Read the model definition and answer for the solid it produces. Units are mm, in the model's axes. A direction names the side the tool comes from. Coordinates: 2 decimals unless noted, no trailing zeros. Order: outer loops, then holes, each group sorted by start corner. A loop starts at its lowest first (then second) coordinate and runs counter-clockwise, first axis right, second up. Notation, with made-up numbers: (43, 84) -> (90, 84) arc R14 ccw to (90, 92) -> close; hole circle Ø2 at (34, 20.5). An arc over 180 degrees is marked (long way). Answer in a Markdown table with one row per item.
from build123d import *

# Parameters (mm, degrees)
CROQUIS1_W              = 19
CROQUIS1_H              = 15
SALIENTE_EXTRUIR1_DEPTH = 7
CROQUIS2_W              = 8
CROQUIS2_H              = 8
CROQUIS2_R              = 1
SALIENTE_EXTRUIR2_DEPTH = 4.9
CROQUIS3_W              = 19
CROQUIS3_H              = 3.8
CORTAR_EXTRUIR1_DEPTH   = 37.9
CROQUIS4_R              = 1
CORTAR_EXTRUIR2_DEPTH   = 51.9


with BuildPart() as part:
    # Croquis1 → Saliente-Extruir1 (new body)
    with BuildSketch(Plane(origin=(0, 0, 0), x_dir=(1, 0, 0), z_dir=(0, 1, 0))):
        Polygon((16.592354246, -24.663454956), (16.592354246, 24.436543518), (8.592354246, 24.436543518), (8.592354246, 14.886544281), (-10.407645754, 14.886544281), (-10.407645754, 24.436543518), (-18.407645754, 24.436543518), (-18.407645754, -24.663454956), (-10.407645754, -24.663454956), (-10.407645754, -15.113455719), (8.592354246, -15.113455719), (8.592354246, -24.663454956), align=None)
        with Locations((-0.907645754, -0.113455719)):
            Rectangle(CROQUIS1_W, CROQUIS1_H, mode=Mode.SUBTRACT)
    extrude(amount=SALIENTE_EXTRUIR1_DEPTH)

    # Croquis2 → Saliente-Extruir2 (add)
    with BuildSketch(Plane(origin=(0, 7, 0), x_dir=(1, 0, 0), z_dir=(0, 1, 0))):
        with Locations((-14.407645754, -0.113455719)):
            Rectangle(CROQUIS2_W, CROQUIS2_H)
        with Locations((-14.407645754, -0.113455719)):
            Circle(CROQUIS2_R, mode=Mode.SUBTRACT)
        with Locations((12.592354246, -0.113455719)):
            Rectangle(CROQUIS2_W, CROQUIS2_H)
        with Locations((12.592354246, -0.113455719)):
            Circle(CROQUIS2_R, mode=Mode.SUBTRACT)
    extrude(amount=SALIENTE_EXTRUIR2_DEPTH)

    # Croquis3 → Cortar-Extruir1 (cut)
    with BuildSketch(Plane.XY.offset(15.113455719)):
        with Locations((-0.907645754, 5.1)):
            Rectangle(CROQUIS3_W, CROQUIS3_H)
    extrude(amount=-CORTAR_EXTRUIR1_DEPTH, mode=Mode.SUBTRACT)

    # Croquis4 → Cortar-Extruir2 (cut)
    with BuildSketch(Plane.XY.offset(24.663454956)):
        with Locations((12.592354246, 3.5)):
            Circle(CROQUIS4_R)
        with Locations((-14.407645754, 3.5)):
            Circle(CROQUIS4_R)
    extrude(amount=-CORTAR_EXTRUIR2_DEPTH, mode=Mode.SUBTRACT)


solid = part.part
Q1. For faces 5 (the face through (-1, 2, 15.113)), 6 (the face through (-14, 7, 14)), 7 (the face through (13, 7, 0)), 8 (the face through (-1, 3.2, 11)), determine the directions among +Z, -Z, +X, -X, +Y, -Y from which every point of the face is accessible in a straight line to the end or side of a thin tool.
Outcome:
| item | result |
|---|---|
| face 5 | +Z, +Y, -Y |
| face 6 | +Z, +X, -X, +Y |
| face 7 | +Y |
| face 8 | +Z, -Z, +Y |
Q2. The part is cut by section C-C (x = -4). Write down the section's boundary in (y, z), then the cut area to 3 significant figures.
Outcome:
| item | result |
|---|---|
| outline | (0, -14.89) -> (3.2, -14.89) -> (3.2, -7.39) -> (0, -7.39) -> close; (0, 7.61) -> (3.2, 7.61) -> (3.2, 15.11) -> (0, 15.11) -> close |
| area | 48.0 mm² |
Q3. The part is cut by section B-B (z = 13.5). Write down the section's boundary in (x, y).
Outcome:
| item | result |
|---|---|
| outline | (-18.41, 0) -> (16.59, 0) -> (16.59, 7) -> (8.59, 7) -> (8.59, 3.2) -> (-10.41, 3.2) -> (-10.41, 7) -> (-18.41, 7) -> close; hole circle Ø2 at (-14.41, 3.5); hole circle Ø2 at (12.59, 3.5) |
Q4. Consider line 1 (X direction, y = 5.5, z = 7); line 2 (X direction, y = 3.25, z = 20.5); line 3 (Y direction, x = -3, z = -7.5). Determine where each line is inside the solid, lowest interval first.
Outcome:
| item | result |
|---|---|
| line 1 | -18.41 to -10.41, 8.59 to 16.59 |
| line 2 | -18.41 to -15.38, -13.44 to -10.41, 8.59 to 11.62, 13.56 to 16.59 |
| line 3 | 0 to 3.2 |
Q5. The part is cut by section D-D (y = 10.75). Write down the section's boundary in (x, z), then the cut area to 3 significant figures.
Outcome:
| item | result |
|---|---|
| outline | (-18.41, -3.89) -> (-10.41, -3.89) -> (-10.41, 4.11) -> (-18.41, 4.11) -> close; (8.59, -3.89) -> (16.59, -3.89) -> (16.59, 4.11) -> (8.59, 4.11) -> close; hole circle Ø2 at (-14.41, 0.11); hole circle Ø2 at (12.59, 0.11) |
| area | 122 mm² |
Q6. The part is cut by section A-A (z = 2.5). Write down the section's boundary in (x, y), then the cut area to 3 significant figures.
Outcome:
| item | result |
|---|---|
| outline | (-18.41, 0) -> (-10.41, 0) -> (-10.41, 11.9) -> (-18.41, 11.9) -> close; (8.59, 0) -> (16.59, 0) -> (16.59, 11.9) -> (8.59, 11.9) -> close; hole circle Ø2 at (-14.41, 3.5); hole circle Ø2 at (12.59, 3.5) |
| area | 184 mm² |
Q7. For a pull along X with two mould halves and no side action, classify faces 1 (the face through (-14, 7, 0)), 2 (the face through (16.592, 3, 0)), 3 (the face through (13.546, 9.416, -0.187)), 4 (the face through (13, 11.9, -1)) as pulls with the +X half, pulls with the -X half, needs draft (parallel to the pull), parting line crosses it, or undercut.
Outcome:
| item | result |
|---|---|
| face 1 | undercut |
| face 2 | pulls with the +X half |
| face 3 | undercut |
| face 4 | needs draft |
Q8. Given pin 1 (2.5 mm diameter, centred on x = 10.5, z = -16, fed in from +Y); pin 2 (1 mm diameter, centred on x = 1.5, y = 1.5, fed in from -Z); pin 3 (1 mm diameter, centred on x = -5, y = 1.5, fed in from +Z), each flat-ended and moving along its own axis, determine where each tip first touches the part or whether it passes through.
Outcome:
| item | result |
|---|---|
| pin 1 | y = 7 |
| pin 2 | z = -14.89 |
| pin 3 | z = 15.11 |
